Autodesk Fusion 360 part; units mm, degrees
sketch "Sketch1" plane through (0, 0, 0) normal (0, 0, 1) x (1, 0, 0)
  line L0 (-71.12, 30.48) -> (106.68, 30.48)
  line L1 (106.68, 30.48) -> (106.68, -102.87)
  line L2 (106.68, -102.87) -> (-71.12, -102.87)
  line L3 (-71.12, -102.87) -> (-71.12, 30.48)
  dimension "d1" = 177.8
  dimension "d2" = 133.35
sketch "Sketch2" plane through (0, 0, 0) normal (0, 0, 1) x (1, 0, 0)
  line L0 (-71.12, 30.48) -> (119.38, 30.48)
  line L1 (119.38, 30.48) -> (119.38, -115.57)
  line L2 (119.38, -115.57) -> (-71.12, -115.57)
  line L3 (-71.12, -115.57) -> (-71.12, 30.48)
  dimension "d23" = 146.05
sketch "Sketch3" plane through (-71.12, 0, 0) normal (-1, 0, 0) x (0, -1, 0)
  line L0 (102.87, 0) -> (115.57, 0)
  line L1 (115.57, 0) -> (115.57, 114.3)
  line L2 (115.57, 114.3) -> (102.87, 114.3)
  line L3 (88.9, 5.08) -> (38.1, 5.08)
  line L4 (38.1, 5.08) -> (38.1, 17.78)
  line L5 (38.1, 17.78) -> (88.9, 17.78)
  line L6 (88.9, 17.78) -> (88.9, 5.08)
  line L7 (102.87, 114.3) -> (102.87, 0)
  dimension "d26" = 12.7
sketch "Sketch4" plane through (0, 0, 0) normal (0, 0, 1) x (1, 0, 0)
  line L0 (-76.2, 63.5) -> (-19.05, 63.5)
  line L1 (-19.05, 63.5) -> (-19.05, -6.35)
  line L2 (-19.05, -6.35) -> (-76.2, -6.35)
  line L3 (-76.2, -6.35) -> (-76.2, 63.5)
  dimension "d29" = 57.15
  dimension "d30" = 69.85
extrude "Extrude13" add sketch "Sketch4" along normal blind 40.005
sketch "Sketch5" plane through (0, 0, 40.005) normal (0, 0, 1) x (-1, 0, 0)
  line L0 (76.2, 6.35) -> (19.05, 6.35)
  line L1 (19.05, 6.35) -> (19.05, -63.5)
  line L2 (19.05, -63.5) -> (76.2, -63.5)
  line L3 (76.2, -63.5) -> (76.2, 6.35)
  line L4 (73.66, -60.96) -> (21.7077, -60.96)
  line L5 (21.7077, -60.96) -> (21.7077, 3.8213)
  line L6 (21.7077, 3.8213) -> (73.66, 3.8213)
  line L7 (73.66, 3.8213) -> (73.66, -60.96)
extrude "Extrude14" cut sketch "Sketch5" against normal blind 38.1 contours L4 L5 L6 L7
sketch "Sketch6" plane through (0, -6.35, 0) normal (0, -1, 0) x (1, 0, 0)
  line L0 (-76.2, 0) -> (-19.05, 0)
  line L1 (-19.05, 0) -> (-19.05, 40.005)
  line L2 (-19.05, 40.005) -> (-76.2, 40.005)
  line L3 (-76.2, 40.005) -> (-76.2, 0)
  line L4 (-22.86, 2.54) -> (-73.66, 2.54)
  line L5 (-73.66, 2.54) -> (-73.66, 15.24)
  line L6 (-73.66, 15.24) -> (-22.86, 15.24)
  line L7 (-22.86, 15.24) -> (-22.86, 2.54)
  dimension "d35" = 50.8
  dimension "d36" = 12.7
extrude "Extrude15" cut sketch "Sketch6" against normal blind 19.9898 contours L4 L5 L6 L7
extrude "Extrude16" cut 1 faces at (-56.7267, -4.6642, 2.54) along direction (0, 0, -1) blind 0.635
extrude "Extrude17" add 1 faces at (-39.7933, -4.6642, 15.24) along direction (0, 0, -1) blind 1.905
extrude "Extrude18" add 1 faces at (-19.05, 40.2167, 13.335) along direction (1, 0, 0) blind 6.35
extrude "Extrude19" cut 1 faces at (-21.7077, 17.7724, 27.305) along direction (1, 0, 0) blind 6.35
extrude "Extrude20" cut 1 faces at (-22.86, -4.6642, 5.715) along direction (1, 0, 0) blind 7.62
extrude "Extrude21" add 1 faces at (-15.24, -4.6642, 5.715) along direction (-1, 0, 0) blind 0.127
extrude "Extrude22" add 1 faces at (-55.0333, 63.5, 13.335) along direction (0, 1, 0) blind 6.35
extrude "Extrude23" cut 1 faces at (-54.2259, 60.96, 27.305) along direction (0, 1, 0) blind 6.35
sketch "Sketch7" plane through (0, 0, 1.905) normal (0, 0, 1) x (-1, 0, 0)
  line L0 (15.367, 6.35) -> (15.367, 3.8213)
  line L1 (15.367, 3.8213) -> (15.3577, 3.8213)
  line L2 (15.3577, 3.8213) -> (15.3577, -67.31)
  line L3 (15.3577, -67.31) -> (73.66, -67.31)
  line L4 (73.66, -67.31) -> (73.66, 6.35)
  line L5 (73.66, 6.35) -> (15.367, 6.35)
  line L6 (73.66, 6.35) -> (15.367, 6.35)
  line L7 (15.367, 6.35) -> (15.367, 2.4713)
  line L8 (15.367, 2.4713) -> (73.66, 2.4713)
  line L9 (73.66, 2.4713) -> (73.66, 6.35)
extrude "Extrude24" add sketch "Sketch7" along normal blind 2.54 contours L0 L4 L5 L6 L7 L8 L9
sketch "Sketch8" plane through (0, 0, 13.335) normal (0, 0, -1) x (1, 0, 0)
  line L0 (-15.367, 3.8213) -> (-15.367, 6.35)
  line L1 (-15.367, 6.35) -> (-73.66, 6.35)
  line L2 (-73.66, 6.35) -> (-73.66, 3.8213)
  line L3 (-73.66, 3.8213) -> (-15.367, 3.8213)
  line L4 (-15.367, 3.8213) -> (-28.067, 3.8213)
  line L5 (-28.067, 3.8213) -> (-28.067, 6.35)
  line L6 (-28.067, 6.35) -> (-15.367, 6.35)
  line L7 (-15.367, 6.35) -> (-15.367, 3.8213)
  dimension "d57" = 12.7
extrude "Extrude25" cut sketch "Sketch8" against normal blind 5.0038 contours L0 L1 L3 L4 L5 L6 L7
Geometry: final body of the model. Coordinates: model frame, mm. A direction names the side the tool comes from. Round coordinates to 2 decimals unless told otherwise and drop trailing zeros. Order: outer loops, then holes, each group sorted by start corner. A loop starts at its lowest first (then second) coordinate and runs counter-clockwise, first axis right, second up. Notation, with made-up numbers: (7, 13) -> (48, 13) arc R11 cw to (48, 32) -> close; hole circle Ø2 at (64, 0.25). An arc over 180 degrees is marked (long way). Put each result on its own line as item: value. Start each with the question number.
Q1. Reachability of faces 4 (the flat face through (-51, -5, 13.335)), 5 (the flat face through (-45, -6.35, 24)), 6 (the flat face through (-45, 67.31, 21)) from +Z, -Z, +X, -X, +Y, -Y: full face, straight path, thin tool, end or side. Return the list, or none.
Q2. Section A-A on x = -54. Return the cut outline in (y, z) (3 decimals).
Q3. First-contact query: pin 1 (2 mm diameter, centred on x = -40.5, y = 49, fed in from +Z) (3 decimals). Flat tip, straight axial feed; report the tip coordinate or a pass-through.
Q4. Line query: probe 1 along X at (y, z) = (52.5, 7.5); probe 2 along Y at (x, z) = (-21, 25.5); probe 3 along Y at (x, z) = (-16.5, 4). Output: solid intervals per line, ascending.
Q5. Section B-B on y = 3. Return the cut outline in (x, z) (3 decimals), and give its area (3 significant figures).
Q6. Pull-direction query (X, two-part tool) for faces 1 (the flat face through (-12.7, 31, 20)), 2 (the flat face through (-75, 32, 40.005)), 3 (the flat face through (-44, -3.821, 29)); classes: +X half, -X half, draft (parallel to the pull), parting line (faces both ways), or undercut.
Ans:
1. face 4: -Y
1. face 5: +Z, -Z, +X, -X, -Y
1. face 6: +Z
2. outline: (-6.35, 0) -> (69.85, 0) -> (69.85, 40.005) -> (67.31, 40.005) -> (67.31, 1.905) -> (-2.471, 1.905) -> (-2.471, 4.445) -> (-6.35, 4.445) -> close; (-6.35, 13.335) -> (-3.821, 13.335) -> (-3.821, 40.005) -> (-6.35, 40.005) -> close
3. pin 1: stops at z = 1.905
4. probe 1: x = -76.2 to -73.66, -15.36 to -12.7
4. probe 2: y = -6.35 to -3.82, 67.31 to 69.85
4. probe 3: y = -6.35 to -2.47, 67.31 to 69.85
5. outline: (-76.2, 0) -> (-12.7, 0) -> (-12.7, 40.005) -> (-15.358, 40.005) -> (-15.358, 1.905) -> (-73.66, 1.905) -> (-73.66, 40.005) -> (-76.2, 40.005) -> close
5. area: 319 mm2
6. face 1: +X half
6. face 2: draft
6. face 3: undercut
